Can you work these out from the model? Positions are in its coordinate system, mm. Face numbers are marked on the shaded views. A direction names the side the tool comes from. Coordinates: 2 decimals unless noted, no trailing zeros. Order: outer loops, then holes, each group sorted by start corner. A loop starts at its lowest first (then second) coordinate and runs counter-clockwise, first axis right, second up. Notation, with made-up numbers: (33.5, -28.5) -> (61.5, -28.5) arc R24 cw to (61.5, -15.5) -> close; hole circle Ø7 at (59.25, 44). An arc over 180 degrees is marked (long way). Use a Markdown table: item, result. Add a question column.
1. For pin 1 Ø1 at (x, z) = (21.5, 1.5) entering from -Y; pin 2 Ø0.8 at (y, z) = (9.5, 1.5) entering from +X; pin 3 Ø1 at (x, z) = (12.5, 1.5) entering from -Y, each with a flat end and sliding along its axis, tell me the tip position at first contact or that it passes through.
2. Suppose I cut it at D-D, the plane x = 20.25. List the corners of the cut face in (y, z) for me.
3. We'd pull the mould along Y, two halves only. Please class the marked faces 6, 7 and 8: pulls with the +Y half, pulls with the -Y half, needs draft (parallel to the pull), parting line crosses it, or undercut.
4. For the marked faces 1, 2, 3, 4 and 5, which set-ups out of +Z, -Z, +X, -X, +Y, -Y let a thin tool reach every point of the face, with its end or its side?
5. Suppose I cut it at B-B, the plane x = 4. List the corners of the cut face in (y, z) for me.
6. Suppose I cut it at C-C, the plane x = 23.5. List the corners of the cut face in (y, z) for me, then the cut area to 3 significant figures.
7. If I drill on line 1 along Y through (x, z) = (21.25, 1.4); line 2 along Y through (x, z) = (27, 1.55); line 3 along Y through (x, z) = (1.5, 0.35), over which ranges is the centre line in solid material (lowest first)? Write a range as from..to.
8. Suppose I cut it at A-A, the plane z = 1.6. List the corners of the cut face in (x, y) for me, then the cut area to 3 significant figures.
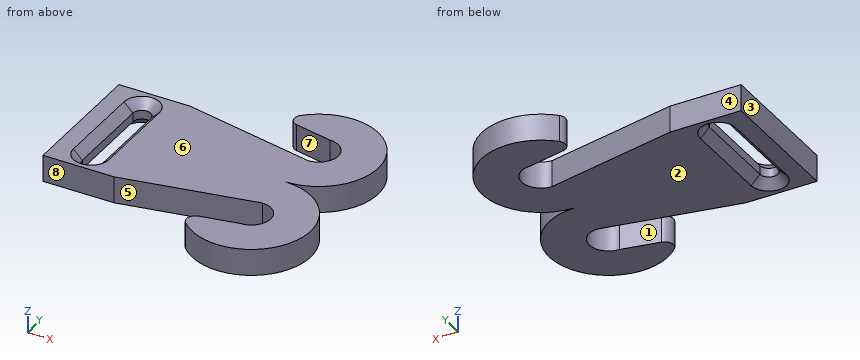
```python
from build123d import *

# Parameters (mm, degrees)
PAD_DEPTH    = 3
POCKET_DEPTH = 5
CHAMFER_SIZE = 1
FILLET_R     = 1


with BuildPart() as part:
    # Sketch → Pad (new body)
    with BuildSketch(Plane.XY):
        with BuildLine():
            Line((0, 15), (0, 0))
            Line((0, 0), (8, 0))
            Line((8, 0), (23, 3))
            ThreePointArc((23, -1.343534), (25.171767, 0.828233), (23, 3))
            Line((23, -1.343534), (17.21767, -2.5))
            ThreePointArc((17.21767, -2.5), (28.775711, -2.511474), (23, 7.5))
            ThreePointArc((23, 7.5), (28.775711, 17.511474), (17.21767, 17.5))
            Line((17.21767, 17.5), (23, 16.343534))
            ThreePointArc((23, 12), (25.171767, 14.171767), (23, 16.343534))
            Line((8, 15), (23, 12))
            Line((0, 15), (8, 15))
        make_face()
    extrude(amount=PAD_DEPTH)

    # Sketch001 (on Face13 of Pad) → Pocket (cut)
    with BuildSketch(Plane.XY.offset(3)):
        with BuildLine():
            ThreePointArc((5, 12.5), (4, 13.5), (3, 12.5))
            Line((3, 12.5), (3, 2.5))
            ThreePointArc((3, 2.5), (4, 1.5), (5, 2.5))
            Line((5, 12.5), (5, 2.5))
        make_face()
    extrude(amount=-POCKET_DEPTH, mode=Mode.SUBTRACT)

    # Chamfer
    chamfer_edges = [part.edges().sort_by_distance(p)[0] for p in [
        (3, 7.5, 0),
        (5, 7.5, 3),
    ]]
    chamfer(chamfer_edges, length=CHAMFER_SIZE)

    # Fillet
    fillet_edges = [part.edges().sort_by_distance(p)[0] for p in [
        (17.21767, -2.5, 1.5),
        (17.21767, 17.5, 1.5),
    ]]
    fillet(fillet_edges, radius=FILLET_R)


solid = part.part
```
Worked out:
| question | item | result |
|---|---|---|
| 1 | pin 1 | stops at y = -5.77 |
| 1 | pin 2 | stops at x = 28.12 |
| 1 | pin 3 | stops at y = 0.8 |
| 2 | outline | (-5.25, 0) -> (-1.89, 0) -> (-1.89, 3) -> (-5.25, 3) -> close; (2.45, 0) -> (12.55, 0) -> (12.55, 3) -> (2.45, 3) -> close; (16.89, 0) -> (20.25, 0) -> (20.25, 3) -> (16.89, 3) -> close |
| 3 | face 6 | needs draft |
| 3 | face 7 | undercut |
| 3 | face 8 | pulls with the -Y half |
| 4 | face 1 | +Z, -Z, -X |
| 4 | face 2 | -Z, +X, -X, +Y, -Y |
| 4 | face 3 | +Z, -Z, -X, +Y, -Y |
| 4 | face 4 | +Z, -Z, -X, +Y |
| 4 | face 5 | +Z, -Z |
| 5 | outline | (0, 0) -> (0.5, 0) -> (1.5, 1) -> (1.5, 2) -> (0.5, 3) -> (0, 3) -> close; (13.5, 1) -> (14.5, 0) -> (15, 0) -> (15, 3) -> (14.5, 3) -> (13.5, 2) -> close |
| 6 | outline | (-5.82, 0) -> (-1.29, 0) -> (-1.29, 3) -> (-5.82, 3) -> close; (2.94, 0) -> (7.48, 0) -> (7.48, 3) -> (2.94, 3) -> close; (7.52, 0) -> (12.06, 0) -> (12.06, 3) -> (7.52, 3) -> close; (16.29, 0) -> (20.82, 0) -> (20.82, 3) -> (16.29, 3) -> close |
| 6 | area | 54.5 mm² |
| 7 | line 1 | y = -5.61..-1.69, 2.65..12.35, 16.69..20.61 |
| 7 | line 2 | y = -4.51..6.17, 8.83..19.51 |
| 7 | line 3 | y = 0..15 |
| 8 | outline | (0, 0) -> (8, 0) -> (23, 3) arc R2.17 cw to (23, -1.34) -> (18.78, -2.19) arc R1 ccw to (18.27, -3.87) arc R6.67 ccw (long way) to (23, 7.5) arc R6.67 ccw (long way) to (18.27, 18.87) arc R1 ccw to (18.78, 17.19) -> (23, 16.34) arc R2.17 cw to (23, 12) -> (8, 15) -> (0, 15) -> close; hole (3, 2.5) arc R1 ccw to (5, 2.5) -> (5, 12.5) arc R1 ccw to (3, 12.5) -> close |
| 8 | area | 435 mm² |
